```python
from build123d import *

# Parameters (mm, degrees)
BOSS_EXTRUDE1_DEPTH         = 6
M6_TAPPED_HOLE1_D           = 5
M6_TAPPED_HOLE1_CSINK_D     = 6.05
M6_TAPPED_HOLE1_CSINK_ANGLE = 90


with BuildPart() as part:
    # Sketch1 → Boss-Extrude1 (new, symmetric)
    with BuildSketch(Plane(origin=(0, 0, 0), x_dir=(0, 0, -1), z_dir=(1, 0, 0))):
        with BuildLine():
            Line((-36, 0), (36, 0))
            Line((36, 0), (36, -31))
            Line((36, -31), (26, -31))
            ThreePointArc((26, -31), (0, -5), (-26, -31))
            Line((-26, -31), (-36, -31))
            Line((-36, -31), (-36, 0))
        make_face()
    extrude(amount=BOSS_EXTRUDE1_DEPTH, both=True)

    # M6 Tapped Hole1 (through all)
    with Locations(Plane(origin=(0, 0, 0), x_dir=(1, 0, 0), z_dir=(0, 1, 0))):
        with Locations((0, -31), (0, 31)):
            CounterSinkHole(M6_TAPPED_HOLE1_D / 2, M6_TAPPED_HOLE1_CSINK_D / 2, counter_sink_angle=M6_TAPPED_HOLE1_CSINK_ANGLE)


solid = part.part
```
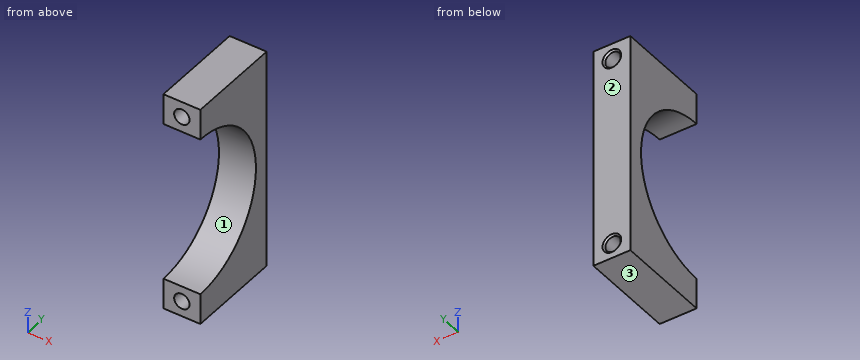
Model file for the job. Use its own axes, mm. Face numbers are marked on the shaded views. Give positions to 0.01 mm unless a question says otherwise; leave off trailing zeros. Order: outer loops, then holes, each group sorted by start corner. A loop starts at its lowest first (then second) coordinate and runs counter-clockwise, first axis right, second up.
1) Saw through at A-A, the plane z = 31. Write the cut outline in (x, y) (3 decimals), then the cut area to 3 significant figures.
2) Mould opens along Z. For the marked faces 1, 2 and 3 say: +Z half, -Z half, draft (parallel to the pull), parting line (faces both ways), or undercut.
3) Saw through at D-D, the plane y = -6.5. Write the cut outline in (x, z).
4) Wall check: probe 1 along X at (y, z) = (-12, 31); probe 2 along Z at (x, y) = (-1, -21); probe 3 along X at (y, z) = (-17, -33). Give the ranges that are in metal, low to high.
5) Saw through at C-C, the plane x = 0. Write the cut outline in (y, z) (3 decimals), then the cut area to 3 significant figures.
6) Pin check, flat tips, straight feed: pin 1 (1 mm diameter, centred on x = 1, z = -1, fed in from -Y); pin 2 (1.5 mm diameter, centred on x = 1, z = -22, fed in from -Y); pin 3 (8 mm diameter, centred on y = -12.5, z = -11.5, fed in from +X). Stop position of each tip, or through.
7) Saw through at B-B, the plane y = -19. Write the cut outline in (x, z), then the cut area to 3 significant figures.
Computed:
1. outline: (-6, -31) - (-2.5, -31) - (-2.5, -0.525) - (-3.025, 0) - (-6, 0) - close; (2.5, -31) - (6, -31) - (6, 0) - (3.025, 0) - (2.5, -0.525) - close
1. area: 217 mm2
2. face 1: undercut
2. face 2: draft
2. face 3: -Z half
3. outline: (-6, -36) - (6, -36) - (6, -8.7) - (-6, -8.7) - close; (-6, 8.7) - (6, 8.7) - (6, 36) - (-6, 36) - close; hole circle Ø5 at (0, -31); hole circle Ø5 at (0, 31)
4. probe 1: x = -6 to -2.5, 2.5 to 6
4. probe 2: z = -36 to -33.29, -28.71 to -24, 24 to 28.71, 33.29 to 36
4. probe 3: x = -6 to -1.5, 1.5 to 6
5. outline: (-31, -36) - (0, -36) - (0, -34.025) - (-0.525, -33.5) - (-31, -33.5) - close; (-31, -28.5) - (-0.525, -28.5) - (0, -27.975) - (0, 27.975) - (-0.525, 28.5) - (-31, 28.5) - (-31, 26) arc R26 cw to (-31, -26) - close; (-31, 33.5) - (-0.525, 33.5) - (0, 34.025) - (0, 36) - (-31, 36) - close
5. area: 860 mm2
6. pin 1: stops at y = -5.04
6. pin 2: stops at y = -18.41
6. pin 3: passes through
7. outline: (-6, -36) - (6, -36) - (6, -23.07) - (-6, -23.07) - close; (-6, 23.07) - (6, 23.07) - (6, 36) - (-6, 36) - close; hole circle Ø5 at (0, -31); hole circle Ø5 at (0, 31)
7. area: 271 mm2
